Answer from the drawing. Dimensions are ordinates in mm from the lowest x, y and z of the part. A direction names the side the tool comes from. Give positions to 0.01 mm unless a question says otherwise; leave off trailing zeros. Order: outer loops, then holes, each group sorted by start corner. A loop starts at its lowest first (then second) coordinate and runs counter-clockwise, first axis right, second up. Notation, with made-up numbers: M 33,-30.5 L 72,-30.5 A21 ccw 72,-26.5 Z; hole C 8.25,-0.75 d1. An arc over 180 degrees is marked long. One line per item, written item: value.
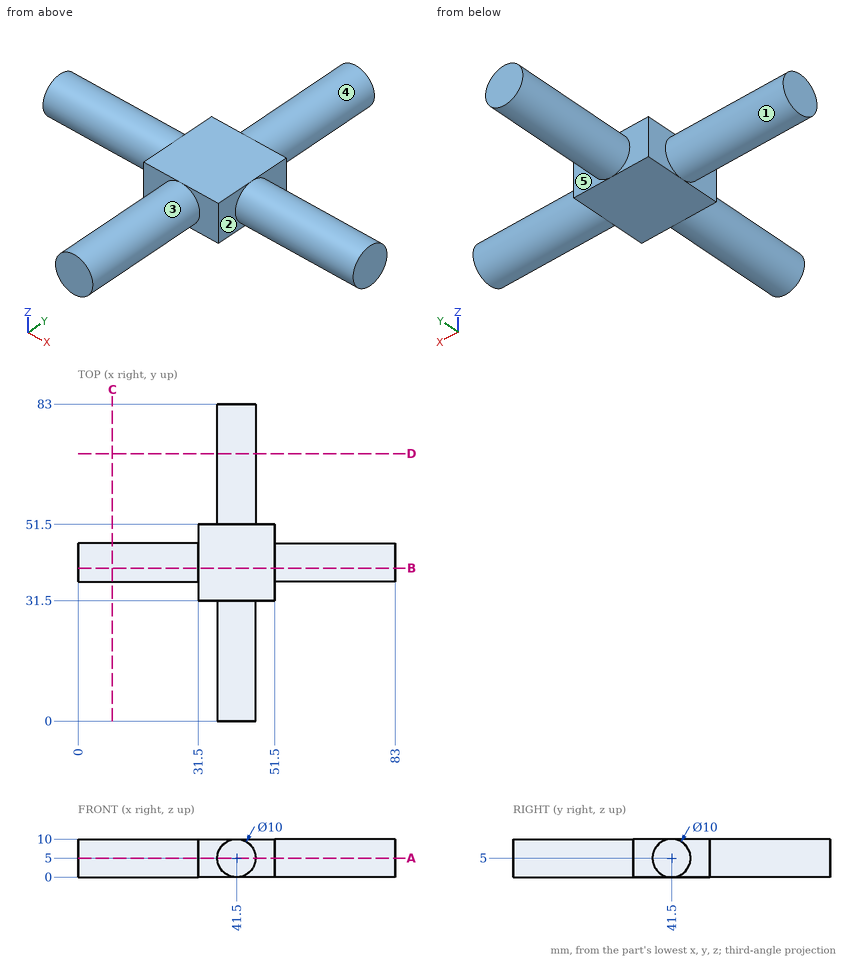
(1) Which of the six approach directions +Z, -Z, +X, -X, +Y, -Y give full straight-line access (tool end or side, diameter ignored) to the marked faces 1, 2, 3, 4 and 5?
Findings:
face 1: -X
face 2: +X, -Y
face 3: -Y
face 4: +Y
face 5: +X, +Y
(2) Given P1, Ø4, axis at x = 28, z = 5, coming from the -Y side, flat-ended and moving along its own axis, determine where the tip first touches the part or whether it passes through.
Findings:
P1: stops at y = 36.5
(3) Section B-B, the plane y = 40 is taken. Give the vertices of the cut face in (x, z).
Findings:
outline: M 0,0.23 L 31.5,0.23 L 31.5,0 L 51.5,0 L 51.5,0.23 L 83,0.23 L 83,9.77 L 51.5,9.77 L 51.5,10 L 31.5,10 L 31.5,9.77 L 0,9.77 Z
(4) Find the intervals of material crossed by probe 1 along Y at (x, z) = (62, 5); probe 2 along Y at (x, z) = (47, 6.5), in increasing order. Write a range as from..to.
Findings:
probe 1: y = 36.5..46.5
probe 2: y = 31.5..51.5
(5) Section A-A, the plane z = 5 is taken. Give the vertices of the cut face in (x, y), then the cut area to 3 significant figures.
Findings:
outline: M 0,36.5 L 31.5,36.5 L 31.5,31.5 L 36.5,31.5 L 36.5,0 L 46.5,0 L 46.5,31.5 L 51.5,31.5 L 51.5,36.5 L 83,36.5 L 83,46.5 L 51.5,46.5 L 51.5,51.5 L 46.5,51.5 L 46.5,83 L 36.5,83 L 36.5,51.5 L 31.5,51.5 L 31.5,46.5 L 0,46.5 Z
area: 1,660 mm^2
(6) Section C-C, the plane x = 9 is taken. Give the vertices of the cut face in (y, z).
Findings:
outline: C 41.5,5 d10
